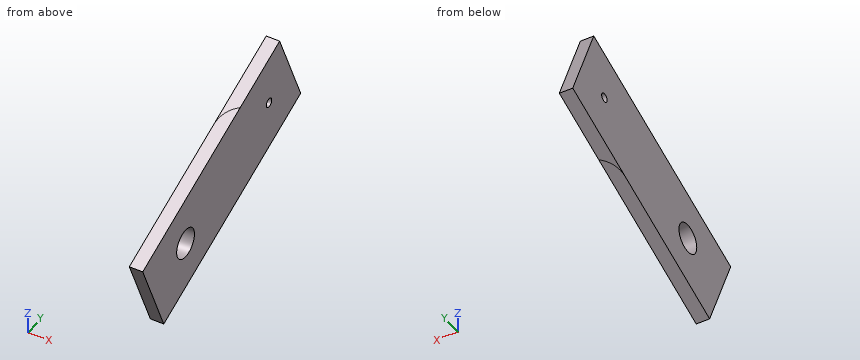
```python
from build123d import *

# Parameters (mm, degrees)
SKETCH1_W                      = 3
SKETCH1_H                      = 40
BOSS_EXTRUDE1_DEPTH            = 20
SKETCH7_R                      = 3.3
M6_CLEARANCE_6_6_MM_THRU_DEPTH = 20
EDGE_FLANGE2_STRIP_W           = 18
EDGE_FLANGE2_STRIP_H           = 3
EDGE_FLANGE2_STRIP_CUT_DEPTH   = 20
EDGE_FLANGE2_DEPTH             = 20
SKETCH21_R                     = 1
CUT_EXTRUDE4_DEPTH             = 10
UNFOLD1_START                  = -35.37712158
UNFOLD1_DEPTH                  = 17
UNFOLD1_START_2                = -38.37712158
UNFOLD1_2_OUTLINE_R            = 1
UNFOLD1_2_DEPTH                = 3


with BuildPart() as part:
    # Sketch1 → Boss-Extrude1 (new body)
    with BuildSketch(Plane(origin=(0, 0.540345249, -1.277454147), x_dir=(-1, 0, 0), z_dir=(0, 0.3895689809965895, -0.9209972904657642))):
        with Locations((36.87712158, 1.824020416)):
            Rectangle(SKETCH1_W, SKETCH1_H)
    extrude(amount=-BOSS_EXTRUDE1_DEPTH)

    # Sketch7 → M6 clearance - 6.6 mm -thru (cut)
    with BuildSketch(Plane.ZY.offset(38.37712158)):
        with Locations((5.916117666, -8.122407734)):
            Circle(SKETCH7_R)
    extrude(amount=-M6_CLEARANCE_6_6_MM_THRU_DEPTH, mode=Mode.SUBTRACT)

    # Edge-Flange2: sheet metal written as solids
    # Edge-Flange2 strip (on a plane across the edge) → Edge-Flange2 strip cut (cut)
    with BuildSketch(Plane(origin=(-35.37712158, 20.640208919, 7.224507248), x_dir=(3.4914813388431334e-15, -0.9209972904657641, -0.3895689809965894), z_dir=(0, -0.3895689809965894, 0.9209972904657641))):
        with Locations((-3, -1.5)):
            Rectangle(EDGE_FLANGE2_STRIP_W, EDGE_FLANGE2_STRIP_H)
    extrude(amount=EDGE_FLANGE2_STRIP_CUT_DEPTH, mode=Mode.SUBTRACT)

    # Edge-Flange2 section (on a plane across the edge) → Edge-Flange2 (add)
    with BuildSketch(Plane(origin=(-35.37712158, 20.640208919, 7.224507248), x_dir=(3.4914813388431334e-15, -0.9209972904657641, -0.3895689809965894), z_dir=(0, -0.3895689809965894, 0.9209972904657641))):
        with BuildLine():
            Line((0, 3), (0, 17))
            Line((0, 17), (3, 17))
            Line((3, 17), (3, 3))
            ThreePointArc((3, 3), (3.878679656, 0.878679656), (6, 0))
            Line((6, 0), (6, -3))
            ThreePointArc((6, -3), (1.757359313, -1.242640687), (0, 3))
        make_face()
    extrude(amount=EDGE_FLANGE2_DEPTH)

    # Sketch21 → Cut-Extrude4 (cut)
    with BuildSketch(Plane(origin=(0, 17.336871798, 7.333254452), x_dir=(-0.3895689809965894, 0.3587919759473664, -0.8482360090452796), z_dir=(3.608224830031759e-15, -0.9209972904657642, -0.3895689809965895))):
        with Locations(Location((2.537974108, -28.109100712, 0), (0, 0, 22.927682802))):
            Circle(SKETCH21_R)
    extrude(amount=-CUT_EXTRUDE4_DEPTH, mode=Mode.SUBTRACT)

    # Unfold1: read off the stored shape, not the designer's step
    # Unfold1 outline → Unfold1 (cut)
    with BuildSketch(Plane.YZ.offset(UNFOLD1_START)):
        Polygon((20.640208919, 7.224507248), (12.848829299, 25.644453057), (7.322845556, 23.307039171), (15.114225176, 4.887093362), align=None)
    extrude(amount=UNFOLD1_DEPTH, mode=Mode.SUBTRACT)

    # Unfold1 2 outline → Unfold1 2 (add)
    with BuildSketch(Plane.YZ.offset(UNFOLD1_START_2)):
        Polygon((34.518333466, 13.094759956), (26.726953846, 31.514705765), (7.322845556, 23.307039171), (15.114225176, 4.887093362), align=None)
        with Locations((22.794166687, 18.993396522)):
            Circle(UNFOLD1_2_OUTLINE_R, mode=Mode.SUBTRACT)
    extrude(amount=UNFOLD1_2_DEPTH)


solid = part.part
```
Geometry check sheet. Reference: the model listing, model coordinates, mm. Coordinates: 2 decimals unless noted, no trailing zeros. Loops run counter-clockwise (first coordinate to the right, second up) from the corner with the lowest first, then second, coordinate; pieces in that order, holes last. Notation, with made-up numbers: (-3, 37) -> (9, 37) arc R19 ccw to (9, 45) -> close; hole circle Ø2 at (33.5, -21.5). An arc over 180 degrees is marked (long way). Put each result on its own line as item: value.
1) Gauge pin test, flat ends, axial feed: pin 1 Ø3 at (y, z) = (22.79, 18.99) entering from -X; pin 2 Ø1.5 at (x, z) = (-36, 14) entering from +Y. Record the tip position at first contact, or that the pin passes through.
Result set:
pin 1: stops at x = -38.38
pin 2: stops at y = 34.45
2) Cross-section at D-D on z = 21.5. Record the boundary of the cut face in (x, y).
Result set:
outline: (-38.38, 3.05) -> (-35.38, 3.05) -> (-35.38, 30.96) -> (-38.38, 30.96) -> close
3) Thickness scan on line 1 (Y direction, x = -37.65, z = 5.5); line 2 (Z direction, x = -35.9, y = -8.5); line 3 (Y direction, x = -36.85, z = 19). Record the ranges inside material, lowest first.
Result set:
line 1: y = -22.06 to -11.4, -4.85 to 16.56
line 2: z = -5.1 to 2.64, 9.19 to 16.61
line 3: y = -2.86 to 21.79, 23.79 to 32.02
4) Cross-section at B-B on z = 6. Record the boundary of the cut face in (x, y), plus the area to 3 significant figures.
Result set:
outline: (-38.38, -22.27) -> (-35.38, -22.27) -> (-35.38, -11.42) -> (-38.38, -11.42) -> close; (-38.38, -4.82) -> (-35.38, -4.82) -> (-35.38, 17.75) -> (-38.38, 17.75) -> close
area: 100 mm^2
5) Cross-section at A-A on y = 23. Record the boundary of the cut face in (x, z).
Result set:
outline: (-38.38, 8.22) -> (-35.38, 8.22) -> (-35.38, 18.01) -> (-38.38, 18.01) -> close; (-38.38, 19.97) -> (-35.38, 19.97) -> (-35.38, 29.94) -> (-38.38, 29.94) -> close
6) Cross-section at C-C on x = -36.2. Record the boundary of the cut face in (y, z).
Result set:
outline: (-23.99, 10.06) -> (-16.2, -8.36) -> (34.52, 13.09) -> (26.73, 31.51) -> close; hole circle Ø6.6 at (-8.12, 5.92); hole circle Ø2 at (22.79, 18.99)
